from build123d import *

# Parameters (mm, degrees)
SKETCH2_W           = 6
SKETCH2_H           = 6
BOSS_EXTRUDE1_DEPTH = 5
SKETCH3_W           = 2
SKETCH3_H           = 4
CUT_EXTRUDE1_DEPTH  = 8
CUT_EXTRUDE2_DEPTH  = 8
SKETCH5_W           = 2
SKETCH5_H           = 4
CUT_EXTRUDE3_DEPTH  = 1


with BuildPart() as part:
    # Sketch2 → Boss-Extrude1 (new body)
    with BuildSketch(Plane(origin=(0, 0, 0), x_dir=(1, 0, 0), z_dir=(0, 1, 0))):
        Rectangle(SKETCH2_W, SKETCH2_H)
    extrude(amount=BOSS_EXTRUDE1_DEPTH)

    # Sketch3 → Cut-Extrude1 (cut)
    with BuildSketch(Plane(origin=(3, 0, 0), x_dir=(0, 0, -1), z_dir=(1, 0, 0))):
        with Locations((2, 3)):
            Rectangle(SKETCH3_W, SKETCH3_H)
    extrude(amount=-CUT_EXTRUDE1_DEPTH, mode=Mode.SUBTRACT)

    # Sketch4 → Cut-Extrude2 (cut)
    with BuildSketch(Plane.XY.offset(3)):
        Polygon((-3, 3), (-1, 5), (-3, 5), align=None)
        Polygon((1, 5), (3, 5), (3, 3), align=None)
    extrude(amount=-CUT_EXTRUDE2_DEPTH, mode=Mode.SUBTRACT)

    # Sketch5 → Cut-Extrude3 (cut)
    with BuildSketch(Plane.XY.offset(3)):
        with Locations((0, 3)):
            Rectangle(SKETCH5_W, SKETCH5_H)
    extrude(amount=-CUT_EXTRUDE3_DEPTH, mode=Mode.SUBTRACT)


solid = part.part
Verification items for the finished model (mm, model axes). A direction names the side the tool comes from. Give positions to 0.01 mm unless a question says otherwise; leave off trailing zeros. Write each loop counter-clockwise with the first axis right and the second up, starting at its lowest first coordinate (ties: lowest second). Pieces come first, ordered by that corner, then holes. Notation, with made-up numbers: M -21.75,45 L 9.25,45 A12 ccw 9.25,57 Z; hole C 25.5,17.25 d1. An arc over 180 degrees is marked long. Write item = value, one per line.
(1) Access from +Z, -Z, +X, -X, +Y, -Y to the whole of each face (thin tool, end or side, straight path). Record for faces 1 (the face through (0, 3, -1)), 2 (the face through (1, 3, 2.5)), 3 (the face through (2, 4, 1)).
Found:
face_1 = -Z, +X, -X, +Y
face_2 = +Z, +Y
face_3 = +Z, -Z, +X, +Y
(2) Sectioned sample at B-B (y = 4.65). Record the cut outline in (x, z), then the cut area to 3 significant figures.
Found:
outline = M -1.35,-1 L 1.35,-1 L 1.35,3 L 1,3 L 1,2 L -1,2 L -1,3 L -1.35,3 Z
area = 8.80 mm2
(3) Go/stop test with flat-tipped pins: pin 1 Ø2 at (x, y) = (0.5, 2.5) entering from -Z; pin 2 Ø0.5 at (x, z) = (-0.5, 2.5) entering from +Y; pin 3 Ø0.8 at (y, z) = (4, 2.5) entering from +X. Record where each tip stops, or that it passes through.
Found:
pin_1 = -1
pin_2 = 1
pin_3 = 2.4
(4) Sectioned sample at D-D (x = -1.1). Record the cut outline in (y, z).
Found:
outline = M 0,-3 L 1,-3 L 1,-1 L 4.9,-1 L 4.9,3 L 0,3 Z
(5) Sectioned sample at C-C (z = -0.1). Record the cut outline in (x, y), then the cut area to 3 significant figures.
Found:
outline = M -3,0 L 3,0 L 3,3 L 1,5 L -1,5 L -3,3 Z
area = 26.0 mm2
(6) Sectioned sample at A-A (x = 0.6). Record the cut outline in (y, z), then the cut area to 3 significant figures.
Found:
outline = M 0,-3 L 1,-3 L 1,-1 L 5,-1 L 5,2 L 1,2 L 1,3 L 0,3 Z
area = 18.0 mm2
(7) Material ranges on line 1 (Y direction, x = 1.7, z = -1.7); line 2 (Z direction, x = -1.4, y = 1.9); line 3 (Z direction, x = -0.6, y = 1.35), recorded low to high.
Found:
line_1 = 0 to 1
line_2 = -1 to 3
line_3 = -1 to 2
